from build123d import *

# Parameters (mm, degrees)
BOSS_EXTRU_1_DEPTH = 10


with BuildPart() as part:
    # Esquisse1 → Boss.-Extru.1 (new body)
    with BuildSketch(Plane(origin=(0, 0, 0), x_dir=(1, 0, 0), z_dir=(0, 1, 0))):
        Polygon((0, 10), (115, 10), (115, 0), (215, 0), (215, 10), (335, 10), (335, 0), (435, 0), (435, 10), (550, 10), (550, 380), (435, 380), (435, 390), (335, 390), (335, 380), (215, 380), (215, 390), (115, 390), (115, 380), (0, 380), align=None)
        Polygon((85, 135), (125, 95), (425, 95), (465, 135), (465, 255), (425, 295), (125, 295), (85, 255), align=None, mode=Mode.SUBTRACT)
    extrude(amount=BOSS_EXTRU_1_DEPTH)


solid = part.part
Verification items for the finished model (mm, model axes). A direction names the side the tool comes from. Give positions to 0.01 mm unless a question says otherwise; leave off trailing zeros. Write each loop counter-clockwise with the first axis right and the second up, starting at its lowest first coordinate (ties: lowest second). Pieces come first, ordered by that corner, then holes.
(1) Cross-section at B-B (z = -268.5). Enter the section's corners in (x, y), plus the area to 3 significant figures.
(2) Cross-section at A-A (x = 457). Enter the section's corners in (y, z).
(3) Mould release check, pull along Z, two halves, no side actions. Record for faces 3 (the face through (445, 5, -275)), 4 (the face through (271, 0, -68)): +Z half, -Z half, draft (parallel to the pull), parting line (faces both ways), or undercut.
(4) Material ranges on line 1 (Z direction, x = 356.5, y = 8.5); line 2 (X direction, y = 6.25, z = -170.5); line 3 (Z direction, x = 288.5, y = 3), recorded low to high.
(5) Access from +Z, -Z, +X, -X, +Y, -Y to the whole of each face (thin tool, end or side, straight path). Record for faces 1 (the face through (271, 10, -68)), 2 (the face through (105, 5, -275)).
(6) Gauge pin test, flat ends, axial feed: pin 1 (5 mm diameter, centred on x = 470.5, y = 3.5, fed in from +Z); pin 2 (3 mm diameter, centred on x = 500.5, y = 6, fed in from -Z); pin 3 (3 mm diameter, centred on y = 3.5, z = -6.5, fed in from +X); pin 4 (6 mm diameter, centred on x = 380.5, y = 2, fed in from +Z). Record the tip position at first contact, or that the pin passes through.
(7) Cross-section at C-C (y = 4.75). Enter the section's corners in (x, z), plus the area to 3 significant figures.
Worked out:
1. outline: (0, 0) - (98.5, 0) - (98.5, 10) - (0, 10) - close; (451.5, 0) - (550, 0) - (550, 10) - (451.5, 10) - close
1. area: 1,970 mm2
2. outline: (0, -380) - (10, -380) - (10, -263) - (0, -263) - close; (0, -127) - (10, -127) - (10, -10) - (0, -10) - close
3. face 3: undercut
3. face 4: draft
4. line 1: z = -390 to -295, -95 to 0
4. line 2: x = 0 to 85, 465 to 550
4. line 3: z = -380 to -295, -95 to -10
5. face 1: +Z, -Z, +X, -X, +Y
5. face 2: +Y, -Y
6. pin 1: stops at z = -10
6. pin 2: stops at z = -380
6. pin 3: stops at x = 435
6. pin 4: stops at z = 0
7. outline: (0, -380) - (115, -380) - (115, -390) - (215, -390) - (215, -380) - (335, -380) - (335, -390) - (435, -390) - (435, -380) - (550, -380) - (550, -10) - (435, -10) - (435, 0) - (335, 0) - (335, -10) - (215, -10) - (215, 0) - (115, 0) - (115, -10) - (0, -10) - close; hole (85, -255) - (125, -295) - (425, -295) - (465, -255) - (465, -135) - (425, -95) - (125, -95) - (85, -135) - close
7. area: 135,000 mm2
